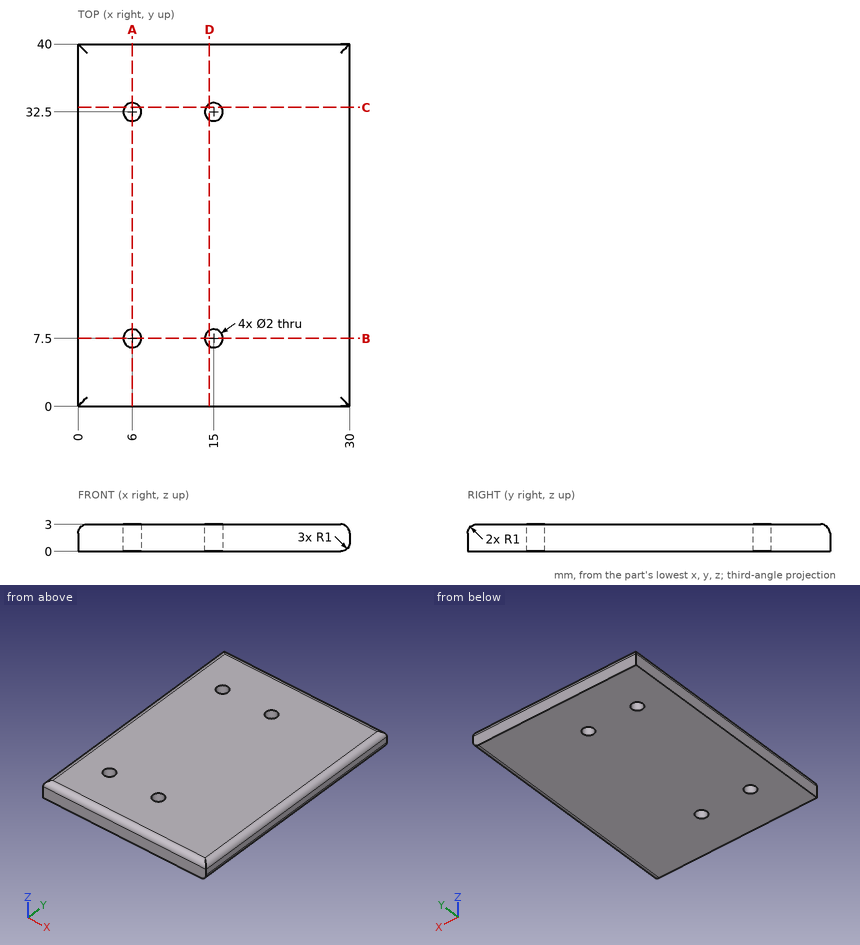
Can you work these out from the drawing? Everything is in mm from the part's minimum corner. Round coordinates to 2 decimals unless told otherwise and drop trailing zeros. Order: outer loops, then holes, each group sorted by start corner. A loop starts at its lowest first (then second) coordinate and runs counter-clockwise, first axis right, second up.
(1) If we section it at C-C (y = 33): Please give me the cut outline in (x, z), plus the area to 3 significant figures.
Results are:
outline: (0, 0) - (5.13, 0) - (5.13, 3) - (1, 3) arc R1 ccw to (0, 2) - close; (6.87, 0) - (14.13, 0) - (14.13, 3) - (6.87, 3) - close; (15.87, 0) - (29, 0) arc R1 ccw to (30, 1) - (30, 2) arc R1 ccw to (29, 3) - (15.87, 3) - close
area: 79.0 mm2
(2) If we section it at D-D (x = 14.5): Please give me the cut outline in (y, z), plus the area to 3 significant figures.
Results are:
outline: (0, 0) - (6.63, 0) - (6.63, 3) - (1, 3) arc R1 ccw to (0, 2) - close; (8.37, 0) - (31.63, 0) - (31.63, 3) - (8.37, 3) - close; (33.37, 0) - (40, 0) - (40, 2) arc R1 ccw to (39, 3) - (33.37, 3) - close
area: 109 mm2
(3) I'm going to push flat-ended pins straight in: pin 1 (12 mm diameter, centred on x = 3.5, y = 28, fed in from -Z); pin 2 (1.6 mm diameter, centred on x = 6, y = 32.5, fed in from +Z). Where does each tip first touch, or does it pass through?
Results are:
pin 1: stops at z = 0
pin 2: passes through
(4) If we section it at A-A (x = 6): Please give me the cut outline in (y, z), plus the area to 3 significant figures.
Results are:
outline: (0, 0) - (6.5, 0) - (6.5, 3) - (1, 3) arc R1 ccw to (0, 2) - close; (8.5, 0) - (31.5, 0) - (31.5, 3) - (8.5, 3) - close; (33.5, 0) - (40, 0) - (40, 2) arc R1 ccw to (39, 3) - (33.5, 3) - close
area: 108 mm2
(5) If I drill on L1, parallel to Y at x = 6, z = 2; L2, parallel to X at y = 32.5, z = 0.9; L3, parallel to Y at x = 14.5, z = 0.55, over which ranges is the centre line in solid material (lowest first)?
Results are:
L1: y = 0 to 6.5, 8.5 to 31.5, 33.5 to 40
L2: x = 0 to 5, 7 to 14, 16 to 29.99
L3: y = 0 to 6.63, 8.37 to 31.63, 33.37 to 40
(6) If we section it at B-B (y = 7.5): Please give me the cut outline in (x, z).
Results are:
outline: (0, 0) - (5, 0) - (5, 3) - (1, 3) arc R1 ccw to (0, 2) - close; (7, 0) - (14, 0) - (14, 3) - (7, 3) - close; (16, 0) - (29, 0) arc R1 ccw to (30, 1) - (30, 2) arc R1 ccw to (29, 3) - (16, 3) - close
